from build123d import *

# Parameters (mm, degrees)
SKETCH1_W           = 3.175
SKETCH1_H           = 25.4
BOSS_EXTRUDE1_DEPTH = 3.175


with BuildPart() as part:
    # Sketch1 → Boss-Extrude1 (new body)
    with BuildSketch(Plane.XY):
        Polygon((65.314285714, 126.5047), (65.214285714, 126.5047), (51.807142857, 126.5047), (51.707142857, 126.5047), (51.707142857, 129.6797), (39.007142857, 129.6797), (39.007142857, 126.5047), (38.907142857, 126.5047), (25.5, 126.5047), (25.4, 126.5047), (25.4, 129.6797), (12.7, 129.6797), (12.7, 126.5047), (12.6, 126.5047), (0, 126.5047), (0, 0), (12.6, 0), (12.7, 0), (12.7, -3.175), (25.4, -3.175), (25.4, 0), (25.5, 0), (38.907142857, 0), (39.007142857, 0), (39.007142857, -3.175), (51.707142857, -3.175), (51.707142857, 0), (51.807142857, 0), (65.214285714, 0), (65.314285714, 0), (65.314285714, -3.175), (78.014285714, -3.175), (78.014285714, 0), (78.114285714, 0), (91.521428571, 0), (91.621428571, 0), (91.621428571, -3.175), (104.321428571, -3.175), (104.321428571, 0), (104.421428571, 0), (117.828571429, 0), (117.928571429, 0), (117.928571429, -3.175), (130.628571429, -3.175), (130.628571429, 0), (130.728571429, 0), (144.135714286, 0), (144.235714286, 0), (144.235714286, -3.175), (156.935714286, -3.175), (156.935714286, 0), (157.035714286, 0), (170.442857143, 0), (170.542857143, 0), (170.542857143, -3.175), (183.242857143, -3.175), (183.242857143, 0), (183.342857143, 0), (196.75, 0), (196.85, 0), (196.85, -3.175), (209.55, -3.175), (209.55, 0), (209.65, 0), (223.057142857, 0), (223.157142857, 0), (223.157142857, -3.175), (235.857142857, -3.175), (235.857142857, 0), (235.957142857, 0), (249.364285714, 0), (249.464285714, 0), (249.464285714, -3.175), (262.164285714, -3.175), (262.164285714, 0), (262.264285714, 0), (275.671428571, 0), (275.771428571, 0), (275.771428571, -3.175), (288.471428571, -3.175), (288.471428571, 0), (288.571428571, 0), (301.978571429, 0), (302.078571429, 0), (302.078571429, -3.175), (314.778571429, -3.175), (314.778571429, 0), (314.878571429, 0), (328.285714286, 0), (328.385714286, 0), (328.385714286, -3.175), (341.085714286, -3.175), (341.085714286, 0), (341.185714286, 0), (354.592857143, 0), (354.692857143, 0), (354.692857143, -3.175), (367.392857143, -3.175), (367.392857143, 0), (367.492857143, 0), (380.9, 0), (381, 0), (381, -3.175), (393.7, -3.175), (393.7, 0), (393.8, 0), (406.4, 0), (406.4, 126.5047), (393.8, 126.5047), (393.7, 126.5047), (393.7, 129.6797), (381, 129.6797), (381, 126.5047), (380.9, 126.5047), (367.492857143, 126.5047), (367.392857143, 126.5047), (367.392857143, 129.6797), (354.692857143, 129.6797), (354.692857143, 126.5047), (354.592857143, 126.5047), (341.185714286, 126.5047), (341.085714286, 126.5047), (341.085714286, 129.6797), (328.385714286, 129.6797), (328.385714286, 126.5047), (328.285714286, 126.5047), (314.878571429, 126.5047), (314.778571429, 126.5047), (314.778571429, 129.6797), (302.078571429, 129.6797), (302.078571429, 126.5047), (301.978571429, 126.5047), (288.571428571, 126.5047), (288.471428571, 126.5047), (288.471428571, 129.6797), (275.771428571, 129.6797), (275.771428571, 126.5047), (275.671428571, 126.5047), (262.264285714, 126.5047), (262.164285714, 126.5047), (262.164285714, 129.6797), (249.464285714, 129.6797), (249.464285714, 126.5047), (249.364285714, 126.5047), (235.957142857, 126.5047), (235.857142857, 126.5047), (235.857142857, 129.6797), (223.157142857, 129.6797), (223.157142857, 126.5047), (223.057142857, 126.5047), (209.65, 126.5047), (209.55, 126.5047), (209.55, 129.6797), (196.85, 129.6797), (196.85, 126.5047), (196.75, 126.5047), (183.342857143, 126.5047), (183.242857143, 126.5047), (183.242857143, 129.6797), (170.542857143, 129.6797), (170.542857143, 126.5047), (170.442857143, 126.5047), (157.035714286, 126.5047), (156.935714286, 126.5047), (156.935714286, 129.6797), (144.235714286, 129.6797), (144.235714286, 126.5047), (144.135714286, 126.5047), (130.728571429, 126.5047), (130.628571429, 126.5047), (130.628571429, 129.6797), (117.928571429, 129.6797), (117.928571429, 126.5047), (117.828571429, 126.5047), (104.421428571, 126.5047), (104.321428571, 126.5047), (104.321428571, 129.6797), (91.621428571, 129.6797), (91.621428571, 126.5047), (91.521428571, 126.5047), (78.114285714, 126.5047), (78.014285714, 126.5047), (78.014285714, 129.6797), (65.314285714, 129.6797), align=None)
        with Locations((401.6375, 88.65235)):
            Rectangle(SKETCH1_W, SKETCH1_H, mode=Mode.SUBTRACT)
        with Locations((401.6375, 37.85235)):
            Rectangle(SKETCH1_W, SKETCH1_H, mode=Mode.SUBTRACT)
        with Locations((4.7625, 88.65235)):
            Rectangle(SKETCH1_W, SKETCH1_H, mode=Mode.SUBTRACT)
        with Locations((4.7625, 37.85235)):
            Rectangle(SKETCH1_W, SKETCH1_H, mode=Mode.SUBTRACT)
    extrude(amount=BOSS_EXTRUDE1_DEPTH)


solid = part.part
Design review of the part built by this model. Coordinates are the model's own, in mm. Give positions to 0.01 mm unless a question says otherwise; leave off trailing zeros. Write each loop counter-clockwise with the first axis right and the second up, starting at its lowest first coordinate (ties: lowest second). Pieces come first, ordered by that corner, then holes. Notation, with made-up numbers: M -14.5,-5.75 L -4.5,-5.75 A23 ccw -4.5,9.25 Z; hole C 73.25,-13.5 d9. An arc over 180 degrees is marked long. Answer as a JSON object with one key per item and string values. Group by question number.
1) We need section A-A (y = 42). Give the boundary of the cut face in (x, z) (3 decimals).
2) For line 1 along X through (y, z) = (83.5, 2.1) (3 decimals); line 2 along Y through (x, z) = (352.5, 2.55), list the stretches that pass through material, from the lowest coordinate up.
3) Clearance check with flat-ended pins moving along their axes: pin 1 Ø1 at (y, z) = (-1.5, 2) entering from +X; pin 2 Ø1 at (x, z) = (244.5, 0.5) entering from +Y; pin 3 Ø1.6 at (y, z) = (128, 1.5) entering from -X. State where each tip first meets the part, or that it passes through.
4) We need section B-B (x = 82). Give the boundary of the cut face in (y, z) (3 decimals).
5) We need section C-C (z = 0.5). Count the separate pieces of the cut face and the enclosed holes in it, and give its area (3 significant figures).
Answer key:
{
 "1": {"outline": "M 0,0 L 3.175,0 L 3.175,3.175 L 0,3.175 Z; M 6.35,0 L 400.05,0 L 400.05,3.175 L 6.35,3.175 Z; M 403.225,0 L 406.4,0 L 406.4,3.175 L 403.225,3.175 Z"},
 "2": {"line 1": "x = 0 to 3.175, 6.35 to 400.05, 403.225 to 406.4", "line 2": "y = 0 to 126.5"},
 "3": {"pin 1": "stops at x = 393.7", "pin 2": "stops at y = 126.5", "pin 3": "stops at x = 12.7"},
 "4": {"outline": "M 0,0 L 126.505,0 L 126.505,3.175 L 0,3.175 Z"},
 "5": {"separate pieces": "1", "enclosed holes": "4", "area": "52,300 mm²"}
}
